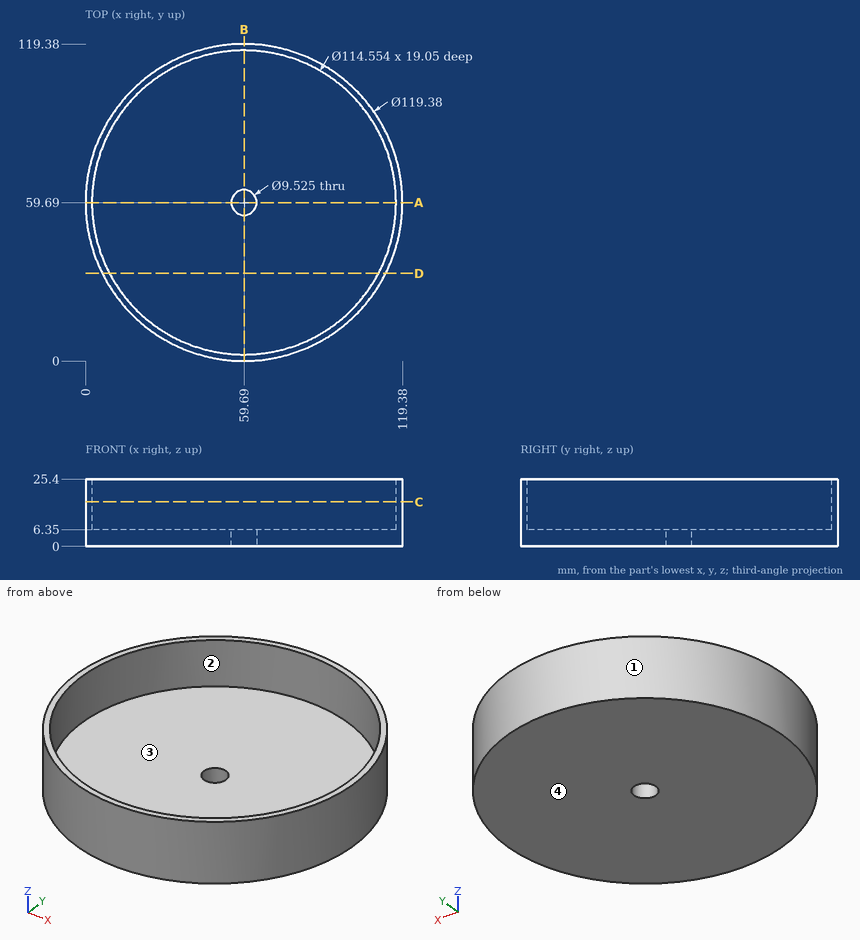
Can you work these out from the drawing? Everything is in mm from the part's minimum corner. Round coordinates to 2 decimals unless told otherwise and drop trailing zeros. Loops run counter-clockwise (first coordinate to the right, second up) from the corner with the lowest first, then second, coordinate; pieces in that order, holes last. Notation, with made-up numbers: M 28,85.5 L 65,85.5 A27 ccw 65,119.5 Z; hole C 65.25,73.5 d11. An arc over 180 degrees is marked long. Write item = value, one per line.
1. Thinking about a two-plate mould opening in X: for the marked faces 1, 2, 3 and 4, which applies, +X half, -X half, draft (parallel to the pull), parting line (faces both ways), or undercut?
Results below:
face_1 = parting line
face_2 = undercut
face_3 = undercut
face_4 = draft
2. Will these pins go through, and if not, where does the flat tip stop? P1, Ø6, axis at y = 96, z = 5, coming from the +X side; P2, Ø6, axis at x = 75, z = 12.5, coming from the +Y side; P3, Ø6, axis at x = 47, z = 4.5, coming from the -Y side.
Results below:
P1 = 109.22
P2 = 118.1
P3 = 0.79
3. I want a section at C-C, the plane z = 16.75. Write out the boundary of the cut face in (x, y), and give its area (3 significant figures).
Results below:
outline = C 59.69,59.69 d119.38; hole C 59.69,59.69 d114.55
area = 887 mm²
4. I want a section at A-A, the plane y = 59.69. Write out the boundary of the cut face in (x, z), and give its area (3 significant figures).
Results below:
outline = M 0,0 L 54.93,0 L 54.93,6.35 L 2.41,6.35 L 2.41,25.4 L 0,25.4 Z; M 64.45,0 L 119.38,0 L 119.38,25.4 L 116.97,25.4 L 116.97,6.35 L 64.45,6.35 Z
area = 790 mm²
5. I need wall thicknesses on probe 1 along Y at (x, z) = (59.69, 14); probe 2 along Y at (x, z) = (59.69, 3.75); probe 3 along Z at (x, y) = (100.5, 90.5). Which ranges of each line are inside material? Lowest first, please.
Results below:
probe_1 = 0 to 2.41, 116.97 to 119.38
probe_2 = 0 to 54.93, 64.45 to 119.38
probe_3 = 0 to 6.35
6. I want a section at D-D, the plane y = 33. Write out the boundary of the cut face in (x, z).
Results below:
outline = M 6.3,0 L 113.08,0 L 113.08,25.4 L 110.37,25.4 L 110.37,6.35 L 9.01,6.35 L 9.01,25.4 L 6.3,25.4 Z
